Geometry check sheet. Reference: the model listing, model coordinates, mm. A direction names the side the tool comes from. Round coordinates to 2 decimals unless told otherwise and drop trailing zeros. Order: outer loops, then holes, each group sorted by start corner. A loop starts at its lowest first (then second) coordinate and runs counter-clockwise, first axis right, second up. Notation, with made-up numbers: (81, 78.5) - (97, 78.5) arc R10 cw to (97, 87.5) - close; hole circle Ø6 at (74, 77). An arc over 180 degrees is marked (long way). Use a Markdown table: item, result. Add a question column.
(1) Section check D-D on y = 0.5. Record the boundary of the cut face in (x, z), then the cut area to 3 significant figures.
(2) Access from +Z, -Z, +X, -X, +Y, -Y to the whole of each face (thin tool, end or side, straight path). Record for faces 5 (the face through (-28.164, 0, 0)), 6 (the face through (0, 4, -23.814)), 7 (the face through (0, -5.5, 22)).
(3) Thickness scan on line 1 along Y through (x, z) = (-4.5, -22); line 2 along Y through (x, z) = (-6.5, 2); line 3 along Z through (x, y) = (14.5, 2.75). Record the ranges inside material, lowest first. Write a range as [from, to].
(4) Section check A-A on y = 8.25. Record the boundary of the cut face in (x, z), then the cut area to 3 significant figures.
(5) Section check C-C on z = 0. Record the boundary of the cut face in (x, y), then the cut area to 3 significant figures.
(6) Section check B-B on x = 0. Record the boundary of the cut face in (y, z).
(7) Mould release check, pull along Z, two halves, no side actions. Record for faces 1 (the face through (0, 0, -26.314)), 2 (the face through (16.7, 8, -29)), 3 (the face through (-0.488, -5.894, -17.804)), 4 (the face through (-0.195, -3.472, -21.487)): released by +Z, released by -Z, zero draft, split by the parting line, or undercut.
(8) Gauge pin test, flat ends, axial feed: P1, Ø2, axis at x = -9, z = -0.5, coming from the +Y side; P2, Ø1.5, axis at x = 6, y = 0.5, coming from the -Z side; P3, Ø2.5, axis at x = -2.5, z = -15.5, coming from the -Y side. Record the tip position at first contact, or that the pin passes through.
Autodesk Inventor part; units mm, degrees
ref_plane "YZ Plane" through (0, 0, 0) normal (1, 0, 0) x (0, 1, 0)
ref_plane "XZ Plane" through (0, 0, 0) normal (0, 1, 0) x (-1, 0, 0)
ref_plane "XY Plane" through (0, 0, 0) normal (0, 0, 1) x (1, 0, 0)
sketch "Sketch1" plane through (0, 0, 0) normal (0, 1, 0) x (-1, 0, 0)
  line L0 (16.85, -26.3137) -> (-16.85, -26.3137)
  line L1 (-16.85, -26.3137) -> (-28.1637, -15)
  line L2 (-28.1637, -15) -> (-28.1637, 15)
  line L3 (-28.1637, 15) -> (-16.85, 26.3137)
  line L4 (-16.85, 26.3137) -> (16.85, 26.3137)
  line L5 (16.85, 26.3137) -> (28.1637, 15)
  line L6 (28.1637, 15) -> (28.1637, -15)
  line L7 (28.1637, -15) -> (16.85, -26.3137)
  point P0 (0, 0)
  point P1 (0, -26.3137)
  point P2 (28.1637, 0)
  point P3 (-28.1637, 0)
  point P4 (0, 26.3137)
  dimension "d2" = 30
  dimension "d6" = 16
  dimension "d7" = 16
  dimension "d9" = 16
  dimension "d10" = 16
  dimension "d11" = 135
  dimension "d12" = 135
  dimension "d13" = 135
  dimension "d14" = 135
  dimension "d15" = 30
  dimension "d16" = 33.7
  dimension "d17" = 33.7
extrude "Extrusion1" add sketch "Sketch1" along normal mid plane 3
sketch "Sketch2" plane through (0, 1.5, 0) normal (0, 1, 0) x (1, 0, 0)
  line L0 (-16.7, 23.8137) -> (16.7, 23.8137)
  line L1 (16.7, 23.8137) -> (16.7, 20.8137)
  line L2 (16.7, 20.8137) -> (-16.7, 20.8137)
  line L3 (-16.7, 20.8137) -> (-16.7, 23.8137)
  line L4 (16.85, 26.3137) -> (-16.85, 26.3137)
  point P0 (0, 0)
  point P1 (0, 23.8137)
  point P2 (0, 26.3137)
  dimension "d20" = 33.4
  dimension "d21" = 3
  dimension "d22" = 2.5
extrude "Extrusion2" add sketch "Sketch2" along normal blind 5.7
sketch "Sketch4" plane through (0, 7.2, 0) normal (0, 1, 0) x (1, 0, 0)
  line L0 (-16.7, 12.2137) -> (16.7, 12.2137)
  line L1 (16.7, 12.2137) -> (16.7, 46.1137)
  line L2 (16.7, 46.1137) -> (-16.7, 46.1137)
  line L3 (-16.7, 46.1137) -> (-16.7, 12.2137)
  line L4 (-16.7, 23.8137) -> (-16.7, 20.8137)
  line L5 (16.7, 20.8137) -> (16.7, 23.8137)
  line L6 (-16.7, 20.8137) -> (16.7, 20.8137)
  line L7 (16.7, 23.8137) -> (-16.7, 23.8137)
  point P0 (0, 0)
  dimension "d25" = 8.6
  dimension "d26" = 22.3
extrude "Extrusion3" add sketch "Sketch4" along normal blind 3
chamfer "Chamfer1" distance 2 angle 45 4 edges at (-16.7, 8.7, -46.1137) (16.7, 8.7, -46.1137) (-16.7, 8.7, -12.2137) (16.7, 8.7, -12.2137)
sketch "Sketch5" plane through (0, -1.5, 0) normal (0, -1, 0) x (1, 0, 0)
  circle A0 centre (0, -20) radius 1.5
  circle A1 centre (0, 20) radius 1.5
  line L0 (-28.1637, -15) -> (-28.1637, 15)
  line L1 (-28.1637, 18.5) -> (28.1637, 18.5)
  line L2 (28.1637, -15) -> (28.1637, 15)
  line L3 (-28.1637, -18.5) -> (28.1637, -18.5)
  line L4 (-28.1637, 21.5) -> (28.1637, 21.5)
  line L5 (-28.1637, -21.5) -> (28.1637, -21.5)
  point P0 (0, 0)
  dimension "d34" = 3
  dimension "d35" = 3
  dimension "d42" = 43
  dimension "d43" = 21.5
  dimension "d44" = 37
  dimension "d45" = 18.5
extrude "Extrusion4" add sketch "Sketch5" along normal blind 4
sketch "Sketch6" plane through (0, -5.5, -20) normal (0, -1, 0) x (1, 0, 0)
  circle A0 centre (0, 0) radius 1.5
  circle A1 centre (0, 0) radius 2.25
  circle A2 centre (0, 40) radius 1.5
  circle A3 centre (0, 40) radius 2.25
  point P0 (0, 20)
  dimension "d38" = 4.5
  dimension "d39" = 4.5
extrude "Extrusion5" add sketch "Sketch6" along normal blind 0.8 contours A0 | A1 | A2 | A3
equation "\"d2\" = d0"
equation "\"d35\" = d34"
equation "\"d39\" = d38"
properties part number "Maker-Bot-Raspberry-Pi-Holder"
Check sheet entries:
| question | item | result |
|---|---|---|
| 1 | outline | (-28.16, -15) - (-16.85, -26.31) - (16.85, -26.31) - (28.16, -15) - (28.16, 15) - (16.85, 26.31) - (-16.85, 26.31) - (-28.16, 15) - close |
| 1 | area | 2,710 mm2 |
| 2 | face 5 | +Z, -Z, -X, +Y, -Y |
| 2 | face 6 | -Z, +X, -X |
| 2 | face 7 | none |
| 3 | line 1 | y = [-1.5, 10.2] |
| 3 | line 2 | y = [-1.5, 1.5] |
| 3 | line 3 | z = [-23.81, -20.81] |
| 4 | outline | (-16.7, -44.11) - (-14.7, -46.11) - (14.7, -46.11) - (16.7, -44.11) - (16.7, -14.21) - (14.7, -12.21) - (-14.7, -12.21) - (-16.7, -14.21) - close |
| 4 | area | 1,120 mm2 |
| 5 | outline | (-28.16, -1.5) - (28.16, -1.5) - (28.16, 1.5) - (-28.16, 1.5) - close |
| 5 | area | 169 mm2 |
| 6 | outline | (-6.3, -22.25) - (-5.5, -22.25) - (-5.5, -21.5) - (-1.5, -21.5) - (-1.5, -26.31) - (1.5, -26.31) - (1.5, -23.81) - (7.2, -23.81) - (7.2, -46.11) - (10.2, -46.11) - (10.2, -12.21) - (7.2, -12.21) - (7.2, -20.81) - (1.5, -20.81) - (1.5, 26.31) - (-1.5, 26.31) - (-1.5, 21.5) - (-5.5, 21.5) - (-5.5, 22.25) - (-6.3, 22.25) - (-6.3, 17.75) - (-5.5, 17.75) - (-5.5, 18.5) - (-1.5, 18.5) - (-1.5, -18.5) - (-5.5, -18.5) - (-5.5, -17.75) - (-6.3, -17.75) - close |
| 7 | face 1 | released by -Z |
| 7 | face 2 | zero draft |
| 7 | face 3 | undercut |
| 7 | face 4 | undercut |
| 8 | P1 | stops at y = 1.5 |
| 8 | P2 | stops at z = -26.31 |
| 8 | P3 | stops at y = -1.5 |
